Autodesk Inventor part; units mm, degrees
ref_plane "YZ Plane" through (0, 0, 0) normal (1, 0, 0) x (0, 1, 0)
ref_plane "XZ Plane" through (0, 0, 0) normal (0, 1, 0) x (-1, 0, 0)
ref_plane "XY Plane" through (0, 0, 0) normal (0, 0, 1) x (1, 0, 0)
sketch "Sketch1" plane through (0, 0, 0) normal (0, 0, 1) x (1, 0, 0)
  line L0 (0, -70.231) -> (0, 54.229)
  line L1 (69.85, 36.449) -> (69.85, -52.451)
  line L2 (69.85, -52.451) -> (-69.85, -52.451)
  line L3 (-69.85, -52.451) -> (-69.85, 36.449)
  line L4 (-97.79, 0) -> (97.79, 0)
  line L5 (-12.7, 36.449) -> (-12.7, 11.049)
  line L6 (-12.7, 11.049) -> (12.7, 11.049)
  line L7 (12.7, 11.049) -> (12.7, 36.449)
  line L8 (-69.85, 36.449) -> (-12.7, 36.449)
  line L9 (12.7, 36.449) -> (69.85, 36.449)
  line L10 (0, -52.451) -> (0, -25.654)
  circle A0 centre (0, -25.654) radius 14.2875
  point P0 (0, 0)
  dimension "d0" = 139.7
  dimension "d1" = 88.9
  dimension "d2" = 25.4
  dimension "d3" = 25.4
  dimension "d5" = 28.575
  dimension "d21" = 62.103
extrude "Extrusion1" add sketch "Sketch1" along normal blind 3.175 contours L2 L3 L4 L0 A0 | L0 A0 L4 L1 L2 | L4 L0 L6 L7 L9 L1 | L3 L8 L5 L6 L0 L4
sketch "Sketch2" plane through (0, 0, 3.175) normal (0, 0, 1) x (1, 0, 0)
  line L0 (69.85, -52.451) -> (69.85, 36.449)
  line L1 (-69.85, -52.451) -> (69.85, -52.451)
  line L2 (69.85, 36.449) -> (12.7, 36.449)
  point P0 (0, 0)
  point P1 (53.975, 17.399)
  point P2 (53.975, -33.401)
  point P3 (53.975, 38.643)
  dimension "d16" = 15.875
  dimension "d18" = 19.05
  dimension "d20" = 19.05
hole "Hole1" at (53.975, 17.399, 3.175) at (53.975, -33.401, 3.175) direction (0, 0, -1) diameter 5.5118 end through all
mirror "Mirror1" about plane through (0, 0, 0) normal (1, 0, 0) of "Hole1"
sketch "Sketch3" plane through (0, 0, 3.175) normal (0, 0, 1) x (1, 0, 0)
  point P0 (0, 0)
properties part number "DIFF_PLATE_ROD"
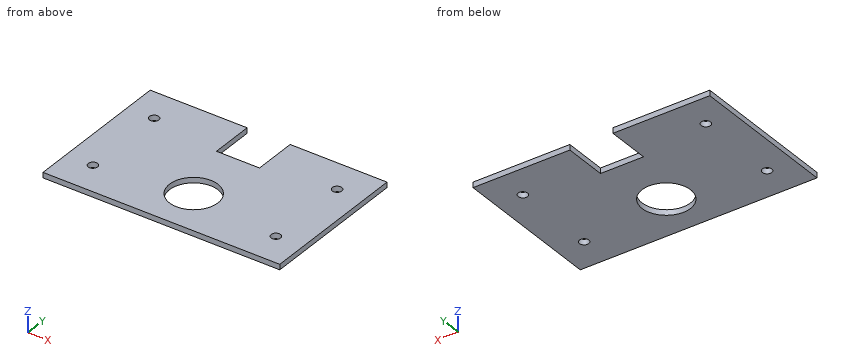
CAD build for the part. Positions are in the model's coordinates, mm. Round coordinates to 2 decimals unless told otherwise and drop trailing zeros. Loops run counter-clockwise (first coordinate to the right, second up) from the corner with the lowest first, then second, coordinate; pieces in that order, holes last. Notation, with made-up numbers: M 11,57 L 56,57 A27 cw 56,95 Z; hole C 8.25,6 d4. An arc over 180 degrees is marked long. Use a Markdown table: item, result. Add a question column.
(1) Drill centre lines: line 1 (X direction, y = 24, z = 1.45); line 2 (Y direction, x = 0, z = 1.15); line 3 (Y direction, x = -55.5, z = 1.55). Where is each one in solid material? Low to high.
(2) Cut at C-C (y = 18). Give the cut face in (x, z) (3 decimals).
(3) Cut at A-A (x = 0). Give the cut face in (y, z) (1 decimal).
(4) Flat gauge pin, fed straight in: pin 1 (1.6 mm diameter, centred on x = -2, z = 2, fed in from +Y). Where does the tip first touch, or does it go through?
(5) Cut at B-B (y = -38). Give the cut face in (x, z) (3 decimals).
(6) Cut at D-D (z = 1.2). State how many separate pieces and enclosed holes the cut face has, and give its area (3 significant figures).
Geometry says:
| question | item | result |
|---|---|---|
| 1 | line 1 | x = -69.85 to -12.7, 12.7 to 69.85 |
| 1 | line 2 | y = -52.45 to -39.94, -11.37 to 11.05 |
| 1 | line 3 | y = -52.45 to -35.7, -31.11 to 15.1, 19.69 to 36.45 |
| 2 | outline | M -69.85,0 L -56.665,0 L -56.665,3.175 L -69.85,3.175 Z; M -51.285,0 L -12.7,0 L -12.7,3.175 L -51.285,3.175 Z; M 12.7,0 L 51.285,0 L 51.285,3.175 L 12.7,3.175 Z; M 56.665,0 L 69.85,0 L 69.85,3.175 L 56.665,3.175 Z |
| 3 | outline | M -52.5,0 L -39.9,0 L -39.9,3.2 L -52.5,3.2 Z; M -11.4,0 L 11,0 L 11,3.2 L -11.4,3.2 Z |
| 4 | pin 1 | stops at y = 11.05 |
| 5 | outline | M -69.85,0 L -7.191,0 L -7.191,3.175 L -69.85,3.175 Z; M 7.191,0 L 69.85,0 L 69.85,3.175 L 7.191,3.175 Z |
| 6 | separate pieces | 1 |
| 6 | enclosed holes | 5 |
| 6 | area | 11,000 mm² |
